Geometry check sheet. Reference: the model listing, model coordinates, mm. A direction names the side the tool comes from. Round coordinates to 2 decimals unless told otherwise and drop trailing zeros. Write each loop counter-clockwise with the first axis right and the second up, starting at its lowest first coordinate (ties: lowest second). Pieces come first, ordered by that corner, then holes. Notation, with made-up numbers: M -23.5,42 L 14.5,42 A8 cw 14.5,52 Z; hole C 74.5,-37.75 d2. An arc over 180 degrees is marked long. Use a Markdown table: item, result.
```python
from build123d import *

# Parameters (mm, degrees)
SKETCH1_R           = 1.5
BOSS_EXTRUDE1_DEPTH = 5
SKETCH2_R           = 2
BOSS_EXTRUDE2_DEPTH = 35


with BuildPart() as part:
    # Sketch1 → Boss-Extrude1 (new body)
    with BuildSketch(Plane(origin=(0, 0, 0), x_dir=(0, 0, -1), z_dir=(1, 0, 0))):
        with BuildLine():
            Line((-5.5, 2), (-5.5, -2))
            Line((-5.5, -2), (5.5, -2))
            Line((5.5, -2), (5.5, 2))
            ThreePointArc((5.5, 2), (0, 7.5), (-5.5, 2))
        make_face()
        with Locations((0, 2)):
            Circle(SKETCH1_R, mode=Mode.SUBTRACT)
    extrude(amount=BOSS_EXTRUDE1_DEPTH)

    # Sketch2 → Boss-Extrude2 (add)
    with BuildSketch(Plane.XZ.offset(2)):
        with Locations(Location((2.5, 0, 0), (0, 0, 270))):
            Circle(SKETCH2_R)
    extrude(amount=BOSS_EXTRUDE2_DEPTH)


solid = part.part
```
Item 1: Cross-section at D-D, the plane z = -3.5. Record the cut outline in (x, y).
Outcome:
| item | result |
|---|---|
| outline | M 0,-2 L 5,-2 L 5,6.24 L 0,6.24 Z |
Item 2: Mould release check, pull along Z, two halves, no side actions. Record for faces 1 (the face through (2.5, 7.5, -0.1)), 2 (the face through (2.465, 0.536, 0.325)), 3 (the face through (2, 0, -5.5)): +Z half, -Z half, draft (parallel to the pull), parting line (faces both ways), or undercut.
Outcome:
| item | result |
|---|---|
| face 1 | parting line |
| face 2 | undercut |
| face 3 | -Z half |
Item 3: Material ranges on line 1 along Y through (x, z) = (3.9, 0); line 2 along Z through (x, y) = (2.45, -22); line 3 along Y through (x, z) = (3.45, -0.75), recorded low to high. Write a range as from..to.
Outcome:
| item | result |
|---|---|
| line 1 | y = -37..0.5, 3.5..7.5 |
| line 2 | z = -2..2 |
| line 3 | y = -37..0.7, 3.3..7.45 |
Item 4: Go/stop test with flat-tipped pins: pin 1 (1 mm diameter, centred on x = 3, z = 1, fed in from +Y); pin 2 (3 mm diameter, centred on x = 3, y = -18, fed in from -Z). Record where each tip stops, or that it passes through.
Outcome:
| item | result |
|---|---|
| pin 1 | stops at y = 7.48 |
| pin 2 | stops at z = -2 |
Item 5: Cross-section at C-C, the plane y = -21.5. Record the cut outline in (x, z).
Outcome:
| item | result |
|---|---|
| outline | C 2.5,0 d4 |
Item 6: Cross-section at B-B, the plane x = 2.5. Record the cut outline in (y, z).
Outcome:
| item | result |
|---|---|
| outline | M -37,-2 L -2,-2 L -2,-5.5 L 2,-5.5 A5.5 ccw 2,5.5 L -2,5.5 L -2,2 L -37,2 Z; hole C 2,0 d3 |
Item 7: Access from +Z, -Z, +X, -X, +Y, -Y to the whole of each face (thin tool, end or side, straight path). Record for faces 4 (the face through (2, 0, 5.5)), 5 (the face through (0.548, -19.255, 0.434)).
Outcome:
| item | result |
|---|---|
| face 4 | +Z, +X, -X, +Y, -Y |
| face 5 | -Y |
Item 8: Cross-section at A-A, the plane z = 0. Record the cut outline in (x, y).
Outcome:
| item | result |
|---|---|
| outline | M 0,-2 L 0.5,-2 L 0.5,-37 L 4.5,-37 L 4.5,-2 L 5,-2 L 5,0.5 L 0,0.5 Z; M 0,3.5 L 5,3.5 L 5,7.5 L 0,7.5 Z |
